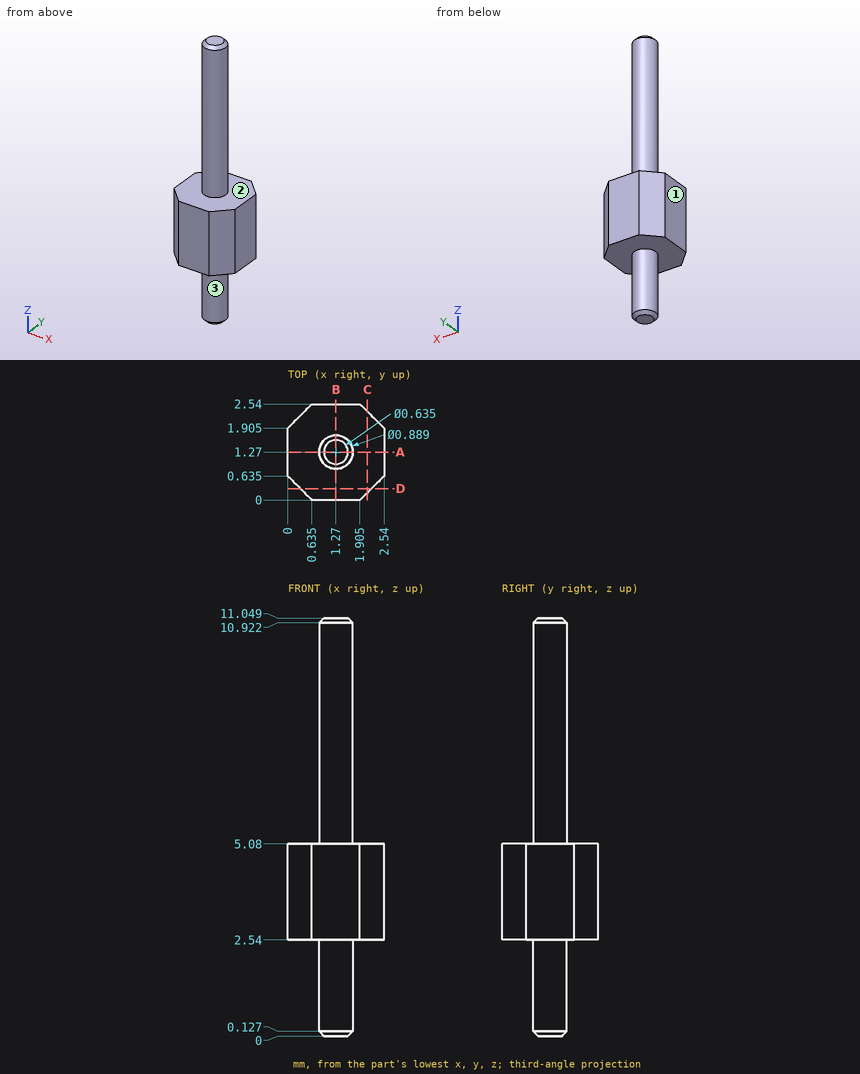
Job drawing, mm, ordinate dimensions from the low corner. One solid piece. A direction names the side the tool comes from. Coordinates: 2 decimals unless noted, no trailing zeros. Order: outer loops, then holes, each group sorted by start corner. A loop starts at its lowest first (then second) coordinate and runs counter-clockwise, first axis right, second up. Notation, with made-up numbers: (70.25, 85) - (75.25, 85) arc R36 cw to (75.25, 121) - close; hole circle Ø10 at (28, 65). An arc over 180 degrees is marked (long way). Write each question's results on one line, items separated by ' | '. Start each with the question number.
Item 1: Tool access for the marked faces 1, 2 and 3: list every direction of +Z, -Z, +X, -X, +Y, -Y with a clear straight run to the whole face (end or side of a thin tool).
Item 2: Wall check: probe 1 along Z at (x, y) = (1, 2.05); probe 2 along Y at (x, z) = (0.45, 4.75) (3 decimals); probe 3 along Z at (x, y) = (1.6, 1.05). Give the ranges that are in metal, low to high. Write a range as [from, to].
Item 3: Flat gauge pins, fed straight in: pin 1 (1.5 mm diameter, centred on x = 1.5, z = 7.5, fed in from -Y); pin 2 (1.5 mm diameter, centred on y = 2, z = 9, fed in from -X). Where does each tip first touch, or does it go through?
Item 4: Band-saw the part on C-C on x = 2.1. Write the cut outline in (y, z) (3 decimals).
Item 5: Band-saw the part on D-D on y = 0.3. Write the cut outline in (x, z) (3 decimals).
Item 6: Band-saw the part on A-A on y = 1.27. Write the cut outline in (x, z), and give its area (3 significant figures).
Numbers:
1) face 1: +Z, -Z, -X, +Y, -Y | face 2: +Z | face 3: -Z
2) probe 1: [2.54, 5.08] | probe 2: [0.185, 2.355] | probe 3: [0.08, 10.97]
3) pin 1: y = 0.83 | pin 2: x = 0.83
4) outline: (0.195, 2.54) - (2.345, 2.54) - (2.345, 5.08) - (0.195, 5.08) - close
5) outline: (0.335, 2.54) - (2.205, 2.54) - (2.205, 5.08) - (0.335, 5.08) - close
6) outline: (0, 2.54) - (0.83, 2.54) - (0.83, 0.13) - (0.95, 0) - (1.59, 0) - (1.71, 0.13) - (1.71, 2.54) - (2.54, 2.54) - (2.54, 5.08) - (1.71, 5.08) - (1.71, 10.92) - (1.59, 11.05) - (0.95, 11.05) - (0.83, 10.92) - (0.83, 5.08) - (0, 5.08) - close | area: 14.0 mm^2
